Can you work these out from the drawing? Everything is in mm from the part's minimum corner. A direction names the side the tool comes from. Give positions to 0.01 mm unless a question says otherwise; leave off trailing zeros. Write each loop counter-clockwise with the first axis right and the second up, starting at its lowest first coordinate (ties: lowest second). Pieces come first, ordered by that corner, then holes. Notation, with made-up numbers: (49, 83) - (74, 83) arc R28 cw to (74, 102) - close; hole circle Ø3 at (-11, 86.5). An arc over 180 degrees is marked (long way). Return JSON: item names as keys, results as strings. Group by question number.
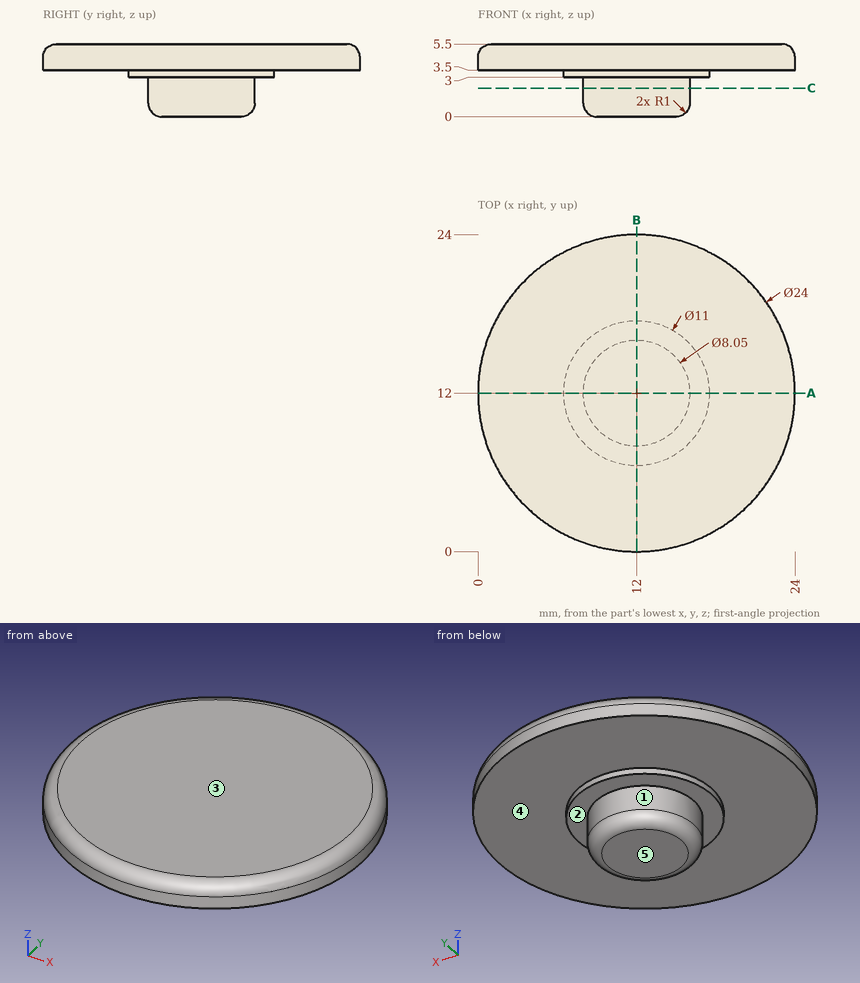
1) I need wall thicknesses on line 1 along Z through (x, y) = (9.75, 1.75); line 2 along Y through (x, z) = (12.25, 3.65); line 3 along Z through (x, y) = (14.25, 8.5). Which ranges of each line are inside material? Lowest first, please.
2) On a 3-axis mill with a long thin cutter (end or side, diameter ignored), from which of +Z, -Z, +X, -X, +Y, -Y can I reach the whole of each face in a straight line? I mean the marked faces 4 and 5. Say none if no direction works.
3) Will these pins go through, and if not, where does the flat tip stop? pin 1 Ø1.5 at (x, z) = (10.5, 3.5) entering from -Y; pin 2 Ø1 at (x, z) = (18.5, 3.5) entering from +Y; pin 3 Ø5.5 at (x, y) = (11.5, 13.5) entering from -Z.
4) Imagine slicing it at A-A, the plane y = 12. Write out the boundary of the cut face in (x, z) (3 decimals), and give its area (3 significant figures).
5) Imagine slicing it at C-C, the plane z = 2.15. Write out the boundary of the cut face in (x, y) (3 decimals), and give its area (3 significant figures).
6) We'd pull the mould along Z, two halves only. Please class the marked faces 1, 2 and 3: pulls with the +Z half, pulls with the -Z half, needs draft (parallel to the pull), parting line crosses it, or undercut.
Resolved:
{
 "1": {"line 1": "3.5 to 5.5", "line 2": "0 to 24", "line 3": "3 to 5.5"},
 "2": {"face 4": "-Z", "face 5": "-Z, +X, -X, +Y, -Y"},
 "3": {"pin 1": "y = 0.02", "pin 2": "y = 22.39", "pin 3": "z = 0"},
 "4": {"outline": "(0, 3.5) - (6.5, 3.5) - (6.5, 3) - (7.975, 3) - (7.975, 1) arc R1 ccw to (8.975, 0) - (15.025, 0) arc R1 ccw to (16.025, 1) - (16.025, 3) - (17.5, 3) - (17.5, 3.5) - (24, 3.5) - (24, 4.5) arc R1 ccw to (23, 5.5) - (1, 5.5) arc R1 ccw to (0, 4.5) - close", "area": "76.8 mm^2"},
 "5": {"outline": "circle Ø8.05 at (12, 12)", "area": "50.9 mm^2"},
 "6": {"face 1": "needs draft", "face 2": "pulls with the -Z half", "face 3": "pulls with the +Z half"}
}
